Could you check a few things on this model? Use its own coordinates, in mm. Face numbers are marked on the shaded views. A direction names the side the tool comes from. Coordinates: 2 decimals unless noted, no trailing zeros. Loops run counter-clockwise (first coordinate to the right, second up) from the corner with the lowest first, then second, coordinate; pieces in that order, holes last. Notation, with made-up numbers: (56, 87) - (111, 87) arc R15 ccw to (111, 107) - close; hole circle Ø10 at (53, -37.5). An arc over 180 degrees is marked (long way). One line per item, written item: value. Start each with the question number.
(1) If we section it at C-C on z = 17: Write out the boundary of the cut face in (x, y).
(2) If we section it at A-A on z = 12.8: Write out the boundary of the cut face in (x, y), then the cut area to 3 significant figures.
(3) I'm going to push flat-ended pins straight in: P1, Ø12, axis at y = 12, z = 10, coming from the +X side; P2, Ø4, axis at x = 17, z = 12, coming from the -Y side; P3, Ø1, axis at x = 8.5, y = 15.5, coming from the +Z side. Where does each tip first touch, or does it pass through?
(4) If we section it at B-B on z = 20.75: Write out the boundary of the cut face in (x, y), then the cut area to 3 significant figures.
(5) If I drill on line 1 along Z through (x, y) = (1.3, 12.8); line 2 along X through (y, z) = (15.75, 17); line 3 along Z through (x, y) = (15.25, 9.5), over which ranges is the centre line in solid material (lowest first)? Write a range as from..to.
(6) If we mould it in two halves opening along X, with no side actions, what happens to the marked faces 1, 2 and 3? For each: pulls with the +X half, pulls with the -X half, needs draft (parallel to the pull), parting line crosses it, or undercut.
(7) On a 3-axis mill with a long thin cutter (end or side, diameter ignored), from which of +Z, -Z, +X, -X, +Y, -Y can I reach the whole of each face in a straight line? I mean the marked faces 4, 5 and 6. Say none if no direction works.
```python
from build123d import *

# Parameters (mm, degrees)
PAD_DEPTH       = 25.4
POCKET_DEPTH    = 23.4
SKETCH002_R     = 7.6
POCKET001_DEPTH = 1.8
FILLET_R        = 1


with BuildPart() as corner:
    # Sketch → Pad (new body)
    with BuildSketch(Plane.XY):
        with BuildLine():
            Line((0, 0), (0, -25.4))
            ThreePointArc((0, -25.4), (15.435414, -20.171961), (24.516737, -6.64))
            Line((0, 0), (24.516737, -6.64))
        make_face()
    extrude(amount=PAD_DEPTH)

    # Sketch001 (on Face5 of Pad) → Pocket (cut)
    with BuildSketch(Plane.XY.offset(25.4)):
        with BuildLine():
            Line((2, -2.5), (2, -27.9))
            ThreePointArc((2, -27.9), (17.435414, -22.671961), (26.516737, -9.14))
            Line((2, -2.5), (26.516737, -9.14))
        make_face()
    extrude(amount=-POCKET_DEPTH, mode=Mode.SUBTRACT)

    # Sketch002 (on Face8 of Pocket) → Pocket001 (cut)
    with BuildSketch(Plane.YZ.offset(2)):
        with Locations((-12.8, 12.8)):
            Circle(SKETCH002_R)
    extrude(amount=-POCKET001_DEPTH, mode=Mode.SUBTRACT)

    # Fillet
    fillet_edges = [corner.edges().sort_by_distance(p)[0] for p in [
        (0, 0, 12.7),
        (12.258369, -3.32, 25.4),
        (24.516737, -6.64, 12.7),
        (12.258369, -3.32, 0),
        (0, -12.7, 0),
        (15.435414, -20.171961, 0),
        (0, -25.4, 12.7),
        (0, -12.7, 25.4),
    ]]
    fillet(fillet_edges, radius=FILLET_R)


with BuildPart() as part_mirroring:
    # Part__Mirroring: instance of Corner
    add(corner.part.mirror(Plane(origin=(0, 0, 0), x_dir=(1, 0, 0), z_dir=(0, 1, 0))))


solid = part_mirroring.part
```
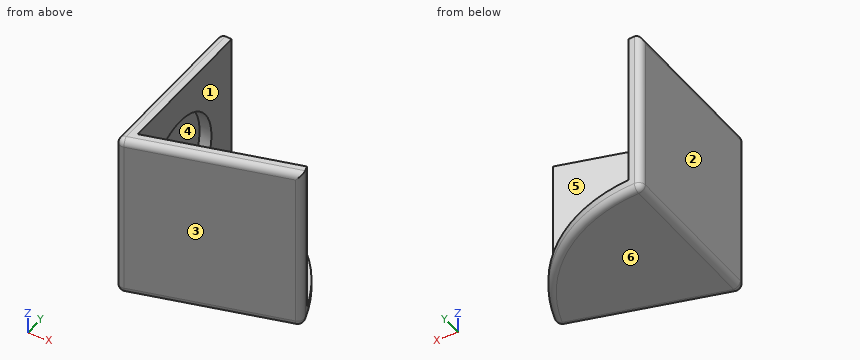
Values:
1. outline: (0, 1.31) arc R1 ccw to (1.26, 0.34) - (23.53, 6.37) arc R1 ccw to (24.22, 7.64) arc R25.4 ccw to (23.95, 8.45) - (2, 2.5) - (2, 6.47) - (0.2, 6.47) - (0.2, 19.13) - (2, 19.13) - (2, 25.32) arc R25.4 ccw to (1.04, 25.38) arc R1 ccw to (0, 24.38) - close
2. outline: (0, 1.31) arc R1 ccw to (1.26, 0.34) - (23.53, 6.37) arc R1 ccw to (24.22, 7.64) arc R25.4 ccw to (23.95, 8.45) - (2, 2.5) - (2, 5.2) - (0.2, 5.2) - (0.2, 20.4) - (2, 20.4) - (2, 25.32) arc R25.4 ccw to (1.04, 25.38) arc R1 ccw to (0, 24.38) - close
2. area: 65.6 mm2
3. P1: stops at x = 24.27
3. P2: stops at y = 4.06
3. P3: stops at z = 2
4. outline: (0, 1.31) arc R1 ccw to (1.26, 0.34) - (23.53, 6.37) arc R1 ccw to (24.22, 7.64) arc R25.4 ccw to (23.95, 8.45) - (2, 2.5) - (2, 25.32) arc R25.4 ccw to (1.04, 25.38) arc R1 ccw to (0, 24.38) - close
4. area: 92.9 mm2
5. line 1: z = 0..5.2, 20.4..25.4
5. line 2: x = 0..0.2
5. line 3: z = 0..2
6. face 1: undercut
6. face 2: pulls with the -X half
6. face 3: pulls with the +X half
7. face 4: none
7. face 5: +Z, +Y
7. face 6: -Z, +X, -X, +Y, -Y
